```python
from build123d import *

# Parameters (mm, degrees)
F0_R      = 1.1
F1_DEPTH  = 1.5
F2_W      = 19.6000001132
F2_H      = 9.6000001132
F3_DEPTH  = 16
F4_W      = 1.5
F4_H      = 4.5
F4_W_2    = 6
F4_H_2    = 5.5
F5_DEPTH  = 1.2
F6_W      = 9
F6_H      = 12
F7_DEPTH  = 25
F8_W      = 16.3223941345
F8_H      = 1
F9_DEPTH  = 1.2
F10_W     = 3
F10_H     = 1.2
F11_DEPTH = 4
F12_W     = 3
F12_H     = 1
F12_W_2   = 2.3728397638
F13_DEPTH = 1.2
F14_W     = 2
F14_H     = 2.5
F14_W_2   = 2.3728397638
F15_DEPTH = 1.2


# Not quite as in the source:
# - a feature names something its author has since deleted; it is built from what else it names


with BuildPart() as f1:
    # F0 (on Top) → F1 (new body)
    with BuildSketch(Plane.XY):
        with BuildLine():
            Line((20.5, 0), (1.5, 0))
            ThreePointArc((1.5, 0), (0.4393398282, -0.4393398282), (0, -1.5))
            Line((0, -1.5), (0, -3.7))
            Line((0, -3.7), (0, -8.3))
            Line((0, -8.3), (0, -10.5))
            ThreePointArc((0, -10.5), (0.4393398282, -11.5606601718), (1.5, -12))
            Line((1.5, -12), (20.5, -12))
            ThreePointArc((20.5, -12), (21.5606601718, -11.5606601718), (22, -10.5))
            Line((22, -10.5), (22, -8.3))
            Line((22, -8.3), (22, -3.7))
            Line((22, -3.7), (22, -1.5))
            ThreePointArc((22, -1.5), (21.5606601718, -0.4393398282), (20.5, 0))
        make_face()
        Polygon((20.8000000566, -1.1999999434), (20.8000000566, -1.5), (20.8000000566, -10.5), (20.8000000566, -10.8000000566), (20.5, -10.8000000566), (1.5, -10.8000000566), (1.1999999434, -10.8000000566), (1.1999999434, -10.5), (1.1999999434, -1.5), (1.1999999434, -1.1999999434), (1.5, -1.1999999434), (20.5, -1.1999999434), align=None, mode=Mode.SUBTRACT)
        with BuildLine():
            Line((0, -8.3), (0, -3.7))
            Line((0, -3.7), (-3.5, -3.7))
            ThreePointArc((-3.5, -3.7), (-4.5606601718, -4.1393398282), (-5, -5.2))
            Line((-5, -5.2), (-5, -6.8))
            ThreePointArc((-5, -6.8), (-4.5606601718, -7.8606601718), (-3.5, -8.3))
            Line((-3.5, -8.3), (0, -8.3))
        make_face()
        with Locations((-2.75, -6)):
            Circle(F0_R, mode=Mode.SUBTRACT)
        with BuildLine():
            Line((25.5, -3.7), (22, -3.7))
            Line((22, -3.7), (22, -8.3))
            Line((22, -8.3), (25.5, -8.3))
            ThreePointArc((25.5, -8.3), (26.5606601718, -7.8606601718), (27, -6.8))
            Line((27, -6.8), (27, -5.2))
            ThreePointArc((27, -5.2), (26.5606601718, -4.1393398282), (25.5, -3.7))
        make_face()
        with Locations((24.75, -6)):
            Circle(F0_R, mode=Mode.SUBTRACT)
    extrude(amount=F1_DEPTH)

    # F2 (on face) → F3 (join)
    with BuildSketch(Plane.XY.offset(1.5)):
        with BuildLine():
            Line((22, -10.5), (22, -8.3))
            Line((22, -8.3), (22, -3.7))
            Line((22, -3.7), (22, -1.5))
            ThreePointArc((22, -1.5), (21.5606601718, -0.4393398282), (20.5, 0))
            Line((20.5, 0), (1.5, 0))
            ThreePointArc((1.5, 0), (0.4393398282, -0.4393398282), (0, -1.5))
            Line((0, -1.5), (0, -3.7))
            Line((0, -3.7), (0, -8.3))
            Line((0, -8.3), (0, -10.5))
            ThreePointArc((0, -10.5), (0.4393398282, -11.5606601718), (1.5, -12))
            Line((1.5, -12), (20.5, -12))
            ThreePointArc((20.5, -12), (21.5606601718, -11.5606601718), (22, -10.5))
        make_face()
        with Locations((11, -6)):
            Rectangle(F2_W, F2_H, mode=Mode.SUBTRACT)
    extrude(amount=F3_DEPTH)

    # F4 (on face) → F5 (cut)
    with BuildSketch(Plane(origin=(0, -10.8000000566, 0), x_dir=(-1, 0, 0), z_dir=(0, 1, 0))):
        with Locations((-20.0500000566, 2.25)):
            Rectangle(F4_W, F4_H)
        Polygon((-16.8000000566, 17.5), (-16.8000000566, 0), (-13.8000000566, 0), (-13.8000000566, 6), (-13.8000000566, 11.5), (-13.8000000566, 17.5), align=None)
        with Locations((-10.8000000566, 8.75)):
            Rectangle(F4_W_2, F4_H_2)
    extrude(amount=-F5_DEPTH, mode=Mode.SUBTRACT)

    # F6 (on face) → F7 (cut)
    with BuildSketch(Plane.XZ.offset(1.1999999434)):
        with Locations((10.9999999434, 6)):
            Rectangle(F6_W, F6_H)
    extrude(amount=-F7_DEPTH, mode=Mode.SUBTRACT)

    # F8 (on face) → F9 (join)
    with BuildSketch(Plane.XY.offset(17.5)):
        with BuildLine():
            Line((16.8000000566, -10.8000000566), (16.8000000566, -12.0000000566))
            Line((16.8000000566, -12), (20.5, -12))
            ThreePointArc((20.5, -12), (21.5606601718, -11.5606601718), (22, -10.5))
            Line((22, -10.5), (22, -1.5))
            ThreePointArc((22, -1.5), (21.5606601718, -0.4393398282), (20.5, 0))
            Line((20.5, 0), (1.5, 0))
            ThreePointArc((1.5, 0), (0.4393398282, -0.4393398282), (0, -1.5))
            Line((0, -1.5), (0, -10.5))
            ThreePointArc((0, -10.5), (0.4393398282, -11.5606601718), (1.5, -12))
            Line((1.5, -12), (13.8000000566, -12))
            Line((13.8000000566, -12.0000000566), (13.8000000566, -10.8000000566))
            Line((13.8000000566, -10.8000000566), (1.1999999434, -10.8000000566))
            Line((1.1999999434, -10.8000000566), (1.1999999434, -1.1999999434))
            Line((1.1999999434, -1.1999999434), (20.8000000566, -1.1999999434))
            Line((20.8000000566, -1.1999999434), (20.8000000566, -10.8000000566))
            Line((20.8000000566, -10.8000000566), (16.8000000566, -10.8000000566))
        make_face()
        Polygon((13.8000000566, -12), (16.8000000566, -12), (16.8000000566, -10.8000000566), (20.8000000566, -10.8000000566), (20.8000000566, -1.1999999434), (1.1999999434, -1.1999999434), (1.1999999434, -10.8000000566), (13.8000000566, -10.8000000566), align=None)
        with Locations((11.0116427531, -9)):
            Rectangle(F8_W, F8_H, mode=Mode.SUBTRACT)
        with Locations((11.0116427531, -7.5)):
            Rectangle(F8_W, F8_H, mode=Mode.SUBTRACT)
        with Locations((11.0116427531, -6)):
            Rectangle(F8_W, F8_H, mode=Mode.SUBTRACT)
        with Locations((11.0116427531, -4.5)):
            Rectangle(F8_W, F8_H, mode=Mode.SUBTRACT)
        with Locations((11.0116427531, -3)):
            Rectangle(F8_W, F8_H, mode=Mode.SUBTRACT)
    extrude(amount=F9_DEPTH)

    # F10 (on face) → F11 (cut)
    with BuildSketch(Plane.XZ.offset(12)):
        with Locations((15.3000000566, 18.1)):
            Rectangle(F10_W, F10_H)
    extrude(amount=-F11_DEPTH, mode=Mode.SUBTRACT)

    # F12 (on face) → F13 (join)
    with BuildSketch(Plane.XY.offset(18.7)):
        with Locations((12.3000000566, -9)):
            Rectangle(F12_W, F12_H)
        with Locations((12.3000000566, -7.5)):
            Rectangle(F12_W, F12_H)
        with Locations((17.9864199385, -7.5)):
            Rectangle(F12_W_2, F12_H)
        with Locations((17.9864199385, -9)):
            Rectangle(F12_W_2, F12_H)
    extrude(amount=-F13_DEPTH)

    # F14 (on face) → F15 (cut)
    with BuildSketch(Plane.XY.offset(18.7)):
        with Locations((12.8000000566, -8.25)):
            Rectangle(F14_W, F14_H)
        with Locations((17.9864199385, -8.25)):
            Rectangle(F14_W_2, F14_H)
    extrude(amount=-F15_DEPTH, mode=Mode.SUBTRACT)


solid = f1.part
```
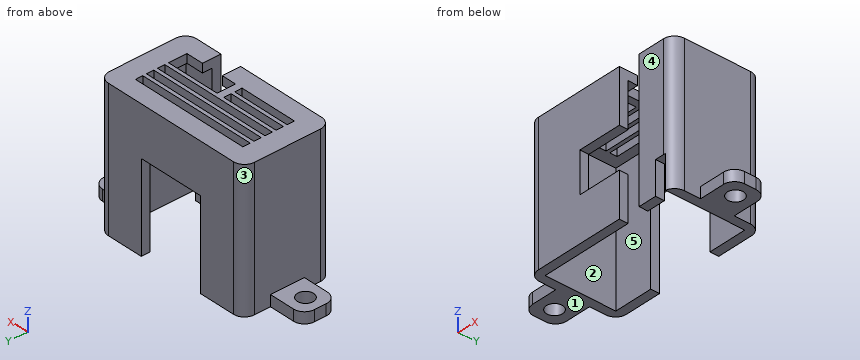
Source: CAD feature listing. Evaluate the final solid. Frame: model axes, mm. Face numbers are marked on the shaded views. A direction names the side the tool comes from. Give positions to 0.01 mm unless a question says otherwise; leave off trailing zeros. Write each loop counter-clockwise with the first axis right and the second up, starting at its lowest first coordinate (ties: lowest second). Pieces come first, ordered by that corner, then holes. Notation, with made-up numbers: (47, -39.75) - (64, -39.75) arc R32 ccw to (64, -1.75) - close; hole circle Ø4 at (71, 32.5). An arc over 180 degrees is marked (long way). One line per item, written item: value. Start each with the question number.
Q1. Section query A-A, the plane z = 2. Return the cut outline in (x, y), then the cut area to 3 significant figures.
Q2. Section query B-B, the plane y = -9. Return the cut outline in (x, z).
Q3. Section query D-D, the plane x = 5.5. Return the cut outline in (y, z).
Q4. Set-up query: the marked faces 1 and 2. Return all of +Z, -Z, +X, -X, +Y, -Y with unobstructed straight access to the full face (end or side cutting, diameter ignored); none if empty.
Q5. Draft query along Y for the marked faces 3, 4 and 5. Return one class per face: +Y half, -Y half, draft (parallel to the pull), parting line (faces both ways), or undercut.
Q6. Material intervals for probe 1 along X at (y, z) = (-8.75, 17.75); probe 2 along Y at (x, z) = (24.75, 1.1); probe 3 along Y at (x, z) = (19, 10), sorted ascending. Write a range as from..to.
Q7. First-contact query: pin 1 Ø1 at (y, z) = (-7.5, 7) entering from +X; pin 2 Ø0.8 at (x, z) = (23, 0.5) entering from -Y; pin 3 Ø7 at (y, z) = (-4.5, 7) entering from -X. Flat tips, straight axial feed; report the tip coordinate or a pass-through.
Q8. Section query C-C, the plane z = 10.5. Return the cut outline in (x, y).
Answer:
1. outline: (0, -10.5) arc R1.5 ccw to (1.5, -12) - (13.8, -12) - (13.8, -10.8) - (1.2, -10.8) - (1.2, -1.2) - (6.5, -1.2) - (6.5, 0) - (1.5, 0) arc R1.5 ccw to (0, -1.5) - close; (15.5, -1.2) - (20.8, -1.2) - (20.8, -11.97) arc R1.5 ccw to (22, -10.5) - (22, -1.5) arc R1.5 ccw to (20.5, 0) - (15.5, 0) - close; (16.8, -12) - (19.3, -12) - (19.3, -10.8) - (16.8, -10.8) - close
1. area: 57.7 mm2
2. outline: (0, 0) - (1.2, 0) - (1.2, 17.5) - (2.85, 17.5) - (2.85, 18.7) - (0, 18.7) - close; (10.8, 17.5) - (11.8, 17.5) - (11.8, 18.7) - (10.8, 18.7) - close; (19.17, 17.5) - (20.8, 17.5) - (20.8, 0) - (22, 0) - (22, 18.7) - (19.17, 18.7) - close
3. outline: (-12, 0) - (-10.8, 0) - (-10.8, 17.5) - (-9.5, 17.5) - (-9.5, 18.7) - (-12, 18.7) - close; (-8.5, 17.5) - (-8, 17.5) - (-8, 18.7) - (-8.5, 18.7) - close; (-7, 17.5) - (-6.5, 17.5) - (-6.5, 18.7) - (-7, 18.7) - close; (-5.5, 17.5) - (-5, 17.5) - (-5, 18.7) - (-5.5, 18.7) - close; (-4, 17.5) - (-3.5, 17.5) - (-3.5, 18.7) - (-4, 18.7) - close; (-2.5, 17.5) - (-1.2, 17.5) - (-1.2, 0) - (0, 0) - (0, 18.7) - (-2.5, 18.7) - close
4. face 1: -Z, +X, -X, +Y, -Y
4. face 2: -Z
5. face 3: +Y half
5. face 4: -Y half
5. face 5: undercut
6. probe 1: x = 0..2.85, 10.8..11.8, 19.17..22
6. probe 2: y = -8.3..-7.1, -4.9..-3.7
6. probe 3: y = -12..-10.8, -1.2..0
7. pin 1: stops at x = 22
7. pin 2: stops at y = -8.3
7. pin 3: stops at x = 0
8. outline: (0, -10.5) arc R1.5 ccw to (1.5, -12) - (7.8, -12) - (7.8, -10.8) - (1.2, -10.8) - (1.2, -1.2) - (6.5, -1.2) - (6.5, 0) - (1.5, 0) arc R1.5 ccw to (0, -1.5) - close; (15.5, -1.2) - (20.8, -1.2) - (20.8, -10.8) - (16.8, -10.8) - (16.8, -12) - (20.5, -12) arc R1.5 ccw to (22, -10.5) - (22, -1.5) arc R1.5 ccw to (20.5, 0) - (15.5, 0) - close
